```python
from build123d import *

# Parameters (mm, degrees)
F0_W     = 320
F0_H     = 320
F0_W_2   = 300
F0_H_2   = 300
F1_DEPTH = 7
F2_DEPTH = 3
F3_R     = 4
F4_DEPTH = 7.5


with BuildPart() as f1:
    # F0 (on Top) → F1 (new body)
    with BuildSketch(Plane.XY):
        Rectangle(F0_W, F0_H)
        Rectangle(F0_W_2, F0_H_2, mode=Mode.SUBTRACT)
        Rectangle(F0_W_2, F0_H_2)
    extrude(amount=F1_DEPTH)

    # F0 (on Top) → F2 (join)
    with BuildSketch(Plane.XY):
        Rectangle(F0_W_2, F0_H_2)
    extrude(amount=-F2_DEPTH)

    # F3 (on Top) → F4 (cut, symmetric)
    with BuildSketch(Plane.XY):
        with Locations((-143, 143)):
            Circle(F3_R)
        with Locations((143, 143)):
            Circle(F3_R)
        with Locations((143, -143)):
            Circle(F3_R)
        with Locations((-143, -143)):
            Circle(F3_R)
    extrude(amount=F4_DEPTH, both=True, mode=Mode.SUBTRACT)


solid = f1.part
```
CAD build for the part. Positions are in the model's coordinates, mm. Round coordinates to 2 decimals unless told otherwise and drop trailing zeros. Write each loop counter-clockwise with the first axis right and the second up, starting at its lowest first coordinate (ties: lowest second). Pieces come first, ordered by that corner, then holes. Notation, with made-up numbers: (70.5, 29) - (120.5, 29) arc R18 ccw to (120.5, 36) - close; hole circle Ø9 at (64, 74). An arc over 180 degrees is marked (long way). Return JSON: item names as keys, results as strings. Group by question number.
Item 1: Flat gauge pins, fed straight in: pin 1 Ø1.5 at (y, z) = (-121, -1) entering from +X; pin 2 Ø0.9 at (x, z) = (-68, -1.5) entering from -Y; pin 3 Ø2.5 at (y, z) = (-8.5, -1.5) entering from -X. Where does each tip first touch, or does it go through?
Item 2: Band-saw the part on C-C on y = 88.5. List the corners of the cut face in (x, z).
Item 3: Mould opens along Y. For faces 1 (the face through (-140.85, -139.627, 2.07)), 2 (the face through (-2, -160, 3)), 3 (the face through (160, -2, 3)) say: +Y half, -Y half, draft (parallel to the pull), parting line (faces both ways), or undercut.
Item 4: Band-saw the part on A-A on x = -143. List the corners of the cut face in (y, z).
Item 5: Probe probe 1 along Y at (x, z) = (-142.5, 0.5); probe 2 along X at (y, z) = (143, 2); probe 3 along X at (y, z) = (-141, 5.5). List the from-to ranges inside material, lowest first.
Resolved:
{
 "1": {"pin 1": "stops at x = 150", "pin 2": "stops at y = -150", "pin 3": "stops at x = -150"},
 "2": {"outline": "(-160, 0) - (-150, 0) - (-150, -3) - (150, -3) - (150, 0) - (160, 0) - (160, 7) - (-160, 7) - close"},
 "3": {"face 1": "undercut", "face 2": "-Y half", "face 3": "draft"},
 "4": {"outline": "(-160, 0) - (-150, 0) - (-150, -3) - (-147, -3) - (-147, 7) - (-160, 7) - close; (-139, -3) - (139, -3) - (139, 7) - (-139, 7) - close; (147, -3) - (150, -3) - (150, 0) - (160, 0) - (160, 7) - (147, 7) - close"},
 "5": {"probe 1": "y = -160 to -146.97, -139.03 to 139.03, 146.97 to 160", "probe 2": "x = -160 to -147, -139 to 139, 147 to 160", "probe 3": "x = -160 to -146.46, -139.54 to 139.54, 146.46 to 160"}
}
